Can you work these out from the model? Positions are in its coordinate system, mm. A direction names the side the tool comes from. Round coordinates to 2 decimals unless told otherwise and drop trailing zeros. Write each loop counter-clockwise with the first axis right and the second up, starting at its lowest first coordinate (ties: lowest second). Pieces come first, ordered by that corner, then holes. Notation, with made-up numbers: (-13, 35) -> (26, 35) arc R14 ccw to (26, 43) -> close; hole circle Ø2 at (13, 46). An arc over 180 degrees is marked (long way). Write item = value, one per line. Start each with the question number.
1) For faces 4 (the face through (45.656, 6, 0)), 5 (the face through (-45.22, -1.2, 0.09)), 6 (the face through (47.78, -2.237, -32.376)), which set-ups out of +Z, -Z, +X, -X, +Y, -Y let a thin tool reach every point of the face, with its end or its side?
2) Thinking about a two-plate mould opening in X: for faces 1 (the face through (-47.78, -2.237, 32.376)), 2 (the face through (-1, 0, 28.972)), 3 (the face through (-1, -2, -33.734)), which applies, +X half, -X half, draft (parallel to the pull), parting line (faces both ways), or undercut?
3) I'm going to push flat-ended pins straight in: pin 1 (0.8 mm diameter, centred on x = -43.5, z = 1.5, fed in from +Y); pin 2 (1.1 mm diameter, centred on x = -45.5, y = 5, fed in from -Z); pin 3 (17.5 mm diameter, centred on x = -20, z = -9.5, fed in from +Y). Where does each tip first touch, or does it pass through?
4) Imagine slicing it at B-B, the plane x = 28. Please give me the cut outline in (y, z), then the cut area to 3 significant figures.
5) If I drill on line 1 (Z direction, x = -40, y = 6.5); line 2 (X direction, y = -1, z = 23); line 3 (Z direction, x = -44, y = 4.25), over which ranges is the centre line in solid material (lowest first)?
6) Imagine slicing it at D-D, the plane z = 3.5. Please give me the cut outline in (x, y).
7) Imagine slicing it at C-C, the plane z = 26. Please give me the cut outline in (x, y).
from build123d import *

# Parameters (mm, degrees)
F1_DEPTH = 7.9375
F3_DEPTH = 4.7625
F5_DEPTH = 6.35


# Not quite as in the source:
# - a pattern or mirror of a feature is missing from the dataset's text; its kind, count and spacing are read off the source's solid


with BuildPart() as f1:
    # F0 (on Front) → F1 (new body, symmetric)
    with BuildSketch(Plane.XZ):
        with BuildLine():
            Line((44.45, 33.734375), (-44.45, 33.734375))
            ThreePointArc((-44.45, 33.734375), (-47.8175960454, 32.3394710454), (-49.2125, 28.971875))
            Line((-49.2125, 28.971875), (-49.2125, -28.971875))
            ThreePointArc((-49.2125, -28.971875), (-47.8175960454, -32.3394710454), (-44.45, -33.734375))
            Line((-44.45, -33.734375), (44.45, -33.734375))
            ThreePointArc((44.45, -33.734375), (47.8175960454, -32.3394710454), (49.2125, -28.971875))
            Line((49.2125, -28.971875), (49.2125, 28.971875))
            ThreePointArc((49.2125, 28.971875), (47.8175960454, 32.3394710454), (44.45, 33.734375))
        make_face()
        with BuildLine():
            ThreePointArc((-42.8625, 27.384375), (-42.3975320151, 28.5069070151), (-41.275, 28.971875))
            Line((-41.275, 28.971875), (41.275, 28.971875))
            ThreePointArc((41.275, 28.971875), (42.3975320151, 28.5069070151), (42.8625, 27.384375))
            Line((42.8625, 27.384375), (42.8625, -27.384375))
            ThreePointArc((42.8625, -27.384375), (42.3975320151, -28.5069070151), (41.275, -28.971875))
            Line((41.275, -28.971875), (-41.275, -28.971875))
            ThreePointArc((-41.275, -28.971875), (-42.3975320151, -28.5069070151), (-42.8625, -27.384375))
            Line((-42.8625, -27.384375), (-42.8625, 27.384375))
        make_face(mode=Mode.SUBTRACT)
    extrude(amount=F1_DEPTH, both=True)

    # F2 (on face) → F3 (join)
    with BuildSketch(Plane.XZ.offset(7.9375)):
        with BuildLine():
            Line((-49.2125, 28.971875), (-49.2125, -28.971875))
            ThreePointArc((-49.2125, -28.971875), (-47.8175960454, -32.3394710454), (-44.45, -33.734375))
            Line((-44.45, -33.734375), (44.45, -33.734375))
            ThreePointArc((44.45, -33.734375), (47.8175960454, -32.3394710454), (49.2125, -28.971875))
            Line((49.2125, -28.971875), (49.2125, 28.971875))
            ThreePointArc((49.2125, 28.971875), (47.8175960454, 32.3394710454), (44.45, 33.734375))
            Line((44.45, 33.734375), (-44.45, 33.734375))
            ThreePointArc((-44.45, 33.734375), (-47.8175960454, 32.3394710454), (-49.2125, 28.971875))
        make_face()
        with BuildLine():
            Line((41.275, -28.971875), (-41.275, -28.971875))
            ThreePointArc((-41.275, -28.971875), (-42.3975320151, -28.5069070151), (-42.8625, -27.384375))
            Line((-42.8625, -27.384375), (-42.8625, 27.384375))
            ThreePointArc((-42.8625, 27.384375), (-42.3975320151, 28.5069070151), (-41.275, 28.971875))
            Line((-41.275, 28.971875), (41.275, 28.971875))
            ThreePointArc((41.275, 28.971875), (42.3975320151, 28.5069070151), (42.8625, 27.384375))
            Line((42.8625, 27.384375), (42.8625, -27.384375))
            ThreePointArc((42.8625, -27.384375), (42.3975320151, -28.5069070151), (41.275, -28.971875))
        make_face(mode=Mode.SUBTRACT)
        with BuildLine():
            ThreePointArc((-42.8625, -27.384375), (-42.3975320151, -28.5069070151), (-41.275, -28.971875))
            Line((-41.275, -28.971875), (41.275, -28.971875))
            ThreePointArc((41.275, -28.971875), (42.3975320151, -28.5069070151), (42.8625, -27.384375))
            Line((42.8625, -27.384375), (42.8625, 27.384375))
            ThreePointArc((42.8625, 27.384375), (42.3975320151, 28.5069070151), (41.275, 28.971875))
            Line((41.275, 28.971875), (-41.275, 28.971875))
            ThreePointArc((-41.275, 28.971875), (-42.3975320151, 28.5069070151), (-42.8625, 27.384375))
            Line((-42.8625, 27.384375), (-42.8625, -27.384375))
        make_face()
    extrude(amount=F3_DEPTH)

    # F4 (on Top) → F5 (cut, symmetric)
    with BuildSketch(Plane.XY):
        with BuildLine():
            Line((-43.9211182963, -1.5875), (-42.8625, -1.5875))
            Line((-42.8625, -1.5875), (-42.8625, 1.5875))
            Line((-42.8625, 1.5875), (-42.8625, 7.9375))
            Line((-42.8625, 7.9375), (-45.6565, 7.9375))
            Line((-45.6565, 7.9375), (-45.6565, 4.8221398621))
            ThreePointArc((-45.6565, 4.8221398621), (-45.712945133, 4.3067430314), (-45.8796045821, 3.8157801263))
            Line((-45.8796045821, 3.8157801263), (-46.4493954179, 2.5938597358))
            ThreePointArc((-46.4493954179, 2.5938597358), (-46.6725, 1.5875), (-46.4493954179, 0.5811402642))
            Line((-46.4493954179, 0.5811402642), (-46.0792637142, -0.2126097358))
            ThreePointArc((-46.0792637142, -0.2126097358), (-45.2005629887, -1.2145758803), (-43.9211182963, -1.5875))
        make_face()
    f5 = extrude(amount=F5_DEPTH, both=True, mode=Mode.SUBTRACT)

    # F5_copies: F5 across plane
    add(f5.mirror(Plane(origin=(0, 0, 0), x_dir=(0, 0, 1), z_dir=(1, 0, 0))), mode=Mode.SUBTRACT)


solid = f1.part
Reported:
q1.face_4 = +Y
q1.face_5 = none
q1.face_6 = -Z, +X, +Y, -Y
q2.face_1 = -X half
q2.face_2 = undercut
q2.face_3 = draft
q3.pin_1 = -1.59
q3.pin_2 = -33.71
q3.pin_3 = -7.94
q4.outline = (-12.7, -33.73) -> (7.94, -33.73) -> (7.94, -28.97) -> (-7.94, -28.97) -> (-7.94, 28.97) -> (7.94, 28.97) -> (7.94, 33.73) -> (-12.7, 33.73) -> close
q4.area = 473 mm²
q5.line_1 = -33.73 to -28.97, 28.97 to 33.73
q5.line_2 = -49.21 to -42.86, 42.86 to 49.21
q5.line_3 = -33.73 to -6.35, 6.35 to 33.73
q6.outline = (-49.21, -12.7) -> (49.21, -12.7) -> (49.21, 7.94) -> (45.66, 7.94) -> (45.66, 4.82) arc R2.38 ccw to (45.88, 3.82) -> (46.45, 2.59) arc R2.38 cw to (46.45, 0.58) -> (46.08, -0.21) arc R2.38 cw to (43.92, -1.59) -> (42.86, -1.59) -> (42.86, -7.94) -> (-42.86, -7.94) -> (-42.86, -1.59) -> (-43.92, -1.59) arc R2.38 cw to (-46.08, -0.21) -> (-46.45, 0.58) arc R2.38 cw to (-46.45, 2.59) -> (-45.88, 3.82) arc R2.38 ccw to (-45.66, 4.82) -> (-45.66, 7.94) -> (-49.21, 7.94) -> close
q7.outline = (-49.21, -12.7) -> (49.21, -12.7) -> (49.21, 7.94) -> (42.86, 7.94) -> (42.86, -7.94) -> (-42.86, -7.94) -> (-42.86, 7.94) -> (-49.21, 7.94) -> close
